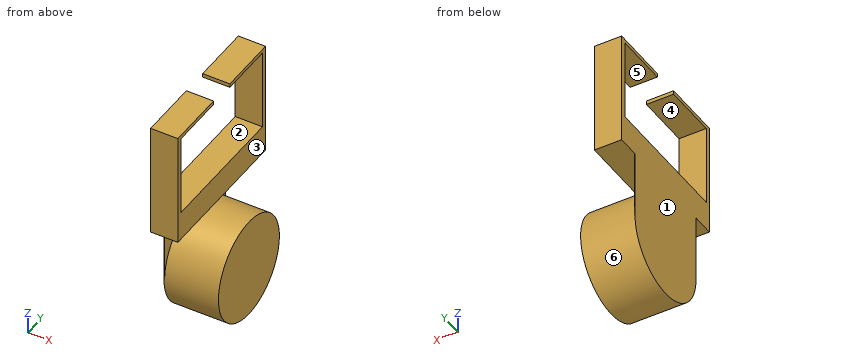
```python
from build123d import *

# Parameters (mm, degrees)
SKETCH1_R           = 23.72487
BOSS_EXTRUDE1_DEPTH = 25.4
SKETCH2_W           = 47.44974
SKETCH2_H           = 0.27178
BOSS_EXTRUDE2_DEPTH = 31.75
SKETCH3_W           = 12.7
SKETCH3_H           = 68.28282
BOSS_EXTRUDE3_DEPTH = 13.65758
SKETCH4_W           = 12.7
SKETCH4_H           = 2.43586
BOSS_EXTRUDE4_DEPTH = 38.0746
SKETCH5_W           = 12.7
SKETCH5_H           = 27.81554
BOSS_EXTRUDE5_DEPTH = 1.77038


with BuildPart() as part:
    # Sketch1 → Boss-Extrude1 (new body)
    with BuildSketch(Plane.YZ):
        with Locations(Location((0, 0, 0), (0, 0, 270))):
            Circle(SKETCH1_R)
    extrude(amount=BOSS_EXTRUDE1_DEPTH)

    # Sketch2 → Boss-Extrude2 (add)
    with BuildSketch(Plane(origin=(0, 0, 0), x_dir=(0, 1, 0), z_dir=(0, 0, 1))):
        with Locations((0, -0.13589)):
            Rectangle(SKETCH2_W, SKETCH2_H)
    extrude(amount=BOSS_EXTRUDE2_DEPTH)

    # Sketch3 → Boss-Extrude3 (add)
    with BuildSketch(Plane.XY.offset(31.75)):
        with Locations((6.35, 0)):
            Rectangle(SKETCH3_W, SKETCH3_H)
    extrude(amount=BOSS_EXTRUDE3_DEPTH)

    # Sketch4 → Boss-Extrude4 (add)
    with BuildSketch(Plane.XY.offset(45.40758)):
        with Locations((6.35, 32.92348)):
            Rectangle(SKETCH4_W, SKETCH4_H)
        with Locations((6.35, -32.92348)):
            Rectangle(SKETCH4_W, SKETCH4_H)
    extrude(amount=BOSS_EXTRUDE4_DEPTH)

    # Sketch5 → Boss-Extrude5 (add)
    with BuildSketch(Plane.XY.offset(83.48218)):
        with Locations((6.35, 20.23364)):
            Rectangle(SKETCH5_W, SKETCH5_H)
        with Locations((6.35, -20.23364)):
            Rectangle(SKETCH5_W, SKETCH5_H)
    extrude(amount=BOSS_EXTRUDE5_DEPTH)


solid = part.part
```
Read the model definition and answer for the solid it produces. Units are mm, in the model's axes. Face numbers are marked on the shaded views. A direction names the side the tool comes from. Coordinates: 2 decimals unless noted, no trailing zeros. Write each loop counter-clockwise with the first axis right and the second up, starting at its lowest first coordinate (ties: lowest second). Pieces come first, ordered by that corner, then holes. Notation, with made-up numbers: (17, 58.5) -> (27, 58.5) arc R12 cw to (27, 75.5) -> close; hole circle Ø11 at (43, 32.5). An arc over 180 degrees is marked (long way). Return JSON: item names as keys, results as strings.
1. A cutting plane is placed at C-C (y = -8.5). Determine the outline of the cut face in (x, z), and give its area (3 significant figures).
Found:
{"outline": "(0, -22.15) -> (25.4, -22.15) -> (25.4, 22.15) -> (0.27, 22.15) -> (0.27, 31.75) -> (12.7, 31.75) -> (12.7, 45.41) -> (0, 45.41) -> close; (0, 83.48) -> (12.7, 83.48) -> (12.7, 85.25) -> (0, 85.25) -> close", "area": "1,320 mm2"}
2. A tool of negligible diameter and unlimited length cuts with its end or side. For the marked faces 1 and 2, from which of +Z, -Z, +X, -X, +Y, -Y can it reach the whole face along a straight path? Write none if from no direction.
Found:
{"face 1": "+Z, -Z, -X, +Y, -Y", "face 2": "+X, -X"}
3. A cutting plane is placed at A-A (x = 4.5). Determine the outline of the cut face in (y, z), and give its area (3 significant figures).
Found:
{"outline": "(-34.14, 31.75) -> (34.14, 31.75) -> (34.14, 85.25) -> (6.33, 85.25) -> (6.33, 83.48) -> (31.71, 83.48) -> (31.71, 45.41) -> (-31.71, 45.41) -> (-31.71, 83.48) -> (-6.33, 83.48) -> (-6.33, 85.25) -> (-34.14, 85.25) -> close; circle Ø47.45 at (0, 0)", "area": "2,980 mm2"}
4. Each of these flat-tipped pins is pushed along its axis until it touches: P1, Ø2, axis at y = -23.5, z = 22.5, coming from the -X side; P2, Ø6, axis at x = 14, z = -5, coming from the -Y side; P3, Ø6, axis at x = 19.5, y = 8, coming from the -Z side; P4, Ø3, axis at x = 19, z = 16, coming from the -Y side. Where does it stop, or does it pass through?
Found:
{"P1": "x = 0", "P2": "y = -23.64", "P3": "z = -23.19", "P4": "y = -18.78"}
5. Determine the mould class of the marked faces 3, 4, 5 and 6 for opening direction Y: pulls with the +Y half, pulls with the -Y half, needs draft (parallel to the pull), parting line crosses it, or undercut.
Found:
{"face 3": "needs draft", "face 4": "undercut", "face 5": "undercut", "face 6": "parting line crosses it"}
6. A cutting plane is placed at B-B (y = 0). Determine the outline of the cut face in (x, z), and give its area (3 significant figures).
Found:
{"outline": "(0, -23.72) -> (25.4, -23.72) -> (25.4, 23.72) -> (0.27, 23.72) -> (0.27, 31.75) -> (12.7, 31.75) -> (12.7, 45.41) -> (0, 45.41) -> close", "area": "1,380 mm2"}
7. Find the intervals of material crossed by line 1 along Z through (x, y) = (7.5, 28); line 2 along Y through (x, z) = (7.75, 77.5); line 3 along Z through (x, y) = (8, 12.5), in increasing order. Write a range as from..to.
Found:
{"line 1": "31.75..45.41, 83.48..85.25", "line 2": "-34.14..-31.71, 31.71..34.14", "line 3": "-20.16..20.16, 31.75..45.41, 83.48..85.25"}
8. A cutting plane is placed at D-D (z = 10). Determine the outline of the cut face in (x, y).
Found:
{"outline": "(0, -23.72) -> (0.27, -23.72) -> (0.27, -21.51) -> (25.4, -21.51) -> (25.4, 21.51) -> (0.27, 21.51) -> (0.27, 23.72) -> (0, 23.72) -> close"}
